Input: part model. Units: mm. Frame: model coordinates. A direction names the side the tool comes from. Give positions to 0.01 mm unless a question says otherwise; leave off trailing zeros. Loops run counter-clockwise (first coordinate to the right, second up) from the corner with the lowest first, then second, coordinate; pieces in that order, holes last. Notation, with made-up numbers: M 33.25,67 L 57.25,67 A14 ccw 57.25,73 Z; hole C 38.25,39.25 d1. An arc over 180 degrees is marked long. Use CSV: the item, a comma, the result in double quotes. Start each with the question number.
Q1. Material intervals for line 1 along X through (y, z) = (2.5, 2); line 2 along Z through (x, y) = (-23, -0.25); line 3 along Y through (x, z) = (-27, -0.5), sorted ascending.
Q2. Pull-direction query (X, two-part tool) for faces 1 (the flat face through (33.7, 2, -2)), 2 (the flat face through (-35.7, 2, -2)), 3 (the cylindrical face through (-0.472, -2.579, 1.978)); classes: released by +X, released by -X, zero draft, split by the parting line, or undercut.
Q3. Reachability of faces 4 (the flat face through (40, 2, -2)), 5 (the cylindrical face through (-39.86, -0.54, 2.44)), 6 (the cylindrical face through (-35.108, -2.579, 1.978)), 7 (the flat face through (34.5, 2, -2)), 8 (the flat face through (-44.3, 0, 0)) from +Z, -Z, +X, -X, +Y, -Y: full face, straight path, thin tool, end or side. Return the list, or none.
Q4. Pin query (flat end, axial travel): pin 1 (2 mm diameter, centred on x = -35.5, y = 2.5, fed in from +Z); pin 2 (2 mm diameter, centred on x = -11, y = -2, fed in from -Z); pin 3 (1.5 mm diameter, centred on x = 4.5, y = -2.5, fed in from +Z). Return the tip coordinate at first contact, or that it passes through.
Q5. Section C-C, the plane x = 9.5. Output: boundary loops of the cut face in (y, z), plus the area to 3 significant figures.
Autodesk Inventor part; units mm, degrees
ref_plane "YZ Plane" through (0, 0, 0) normal (1, 0, 0) x (0, 1, 0)
ref_plane "XZ Plane" through (0, 0, 0) normal (0, 1, 0) x (-1, 0, 0)
ref_plane "XY Plane" through (0, 0, 0) normal (0, 0, 1) x (1, 0, 0)
sketch "Skizze1" plane through (0, 0, 0) normal (0, 0, 1) x (1, 0, 0)
  line L0 (-44.3, 0) -> (44.3, 0)
  line L1 (44.3, 0) -> (44.3, 2.5)
  line L2 (44.3, 2.5) -> (40, 2.5)
  line L3 (40, 2.5) -> (40, 3.25)
  line L4 (33.7, 3.25) -> (-33.7, 3.25)
  line L5 (-35.7, 3.25) -> (-35.7, 2.5)
  line L6 (-35.7, 2.5) -> (-44.3, 2.5)
  line L7 (-44.3, 2.5) -> (-44.3, 0)
  line L8 (0, 3.9) -> (0, -0.65)
  line L9 (-39.8, 2.5) -> (-39.8, 0) construction
  line L10 (-33.7, 3.25) -> (-33.7, 2.5)
  line L11 (-33.7, 2.5) -> (-34.5, 2.5)
  line L12 (-34.5, 2.5) -> (-34.5, 3.25)
  line L13 (-34.5, 3.25) -> (-35.7, 3.25)
  line L14 (33.7, 3.25) -> (33.7, 2.5)
  line L15 (33.7, 2.5) -> (34.5, 2.5)
  line L16 (34.5, 2.5) -> (34.5, 3.25)
  line L17 (34.5, 3.25) -> (40, 3.25)
  point P0 (0, 0)
  dimension "d1" = 4.3
  dimension "d2" = 5
  dimension "d4" = 6.5
  dimension "d18" = 5
  dimension "d20" = 79.8
  dimension "d22" = 4.1
  dimension "d23" = 4.5
  dimension "d24" = 1.2
  dimension "d25" = 0.8
  dimension "d26" = 5
revolve "Umdrehung1" add sketch "Skizze1" angle 360 about axis through (-44.3, 0, 0) along (1, 0, 0)
chamfer "Fase2" distance 0.4 angle 15 1 edges at (-44.3, -2.5, 0) measured on face at (-41.4333, 2.4676, -0.401)
chamfer "Fase3" distance 0.4 angle 15 1 edges at (44.3, -2.5, 0) measured on face at (41.4333, 2.4676, -0.401)
properties part number "Dribblingwelle" material "Aluminium 6061"
A:
1,line 1,"-35.7 to -34.5, -33.7 to 33.7, 34.5 to 40"
1,line 2,"-3.24 to 3.24"
1,line 3,"-3.21 to 3.21"
2,face 1,"undercut"
2,face 2,"released by -X"
2,face 3,"zero draft"
3,face 4,"+X"
3,face 5,"-X"
3,face 6,"+X, -X"
3,face 7,"none"
3,face 8,"+Z, -Z, -X, +Y, -Y"
4,pin 1,"z = 2.88"
4,pin 2,"z = -3.09"
4,pin 3,"z = 2.74"
5,outline,"C 0,0 d6.5"
5,area,"33.2 mm^2"
